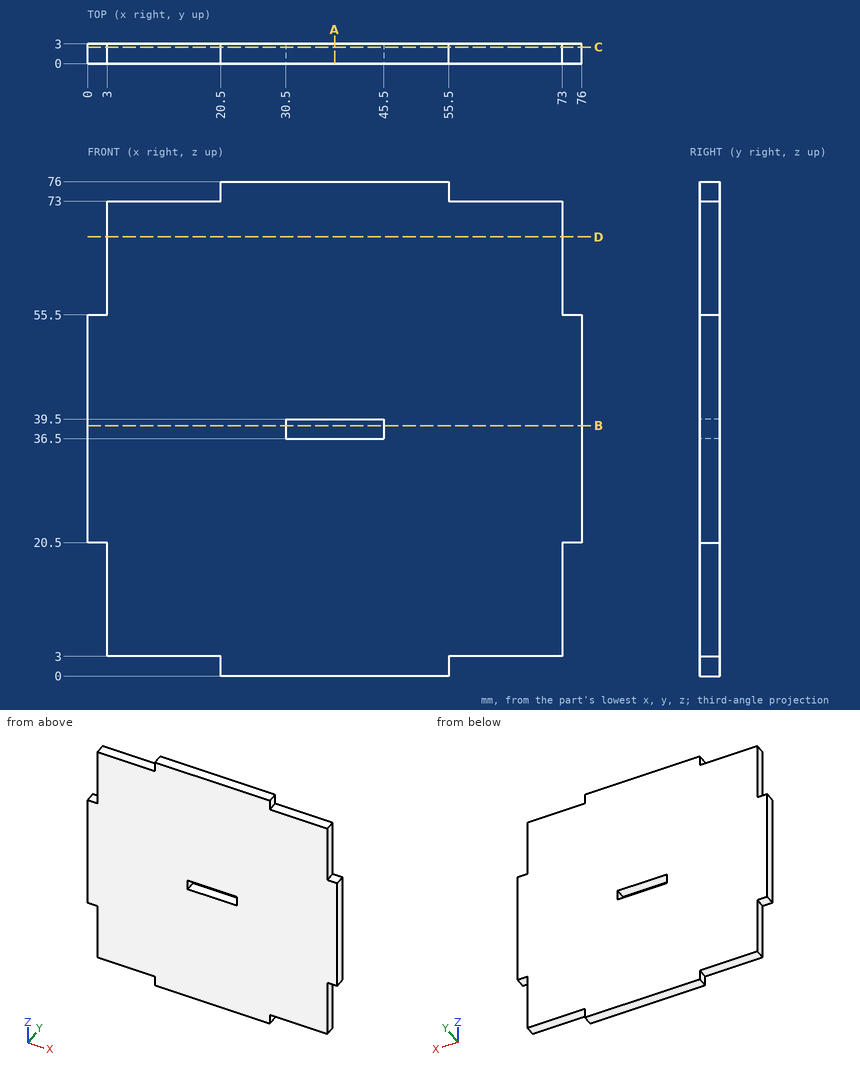
The figure shows three views and two pictorial views of one solid part (mm, origin at its lowest corner). Answer the questions. Give positions to 0.01 mm unless a question says otherwise; leave off trailing zeros. Order: outer loops, then holes, each group sorted by start corner. A loop starts at its lowest first (then second) coordinate and runs counter-clockwise, first axis right, second up. Notation, with made-up numbers: (57, 36.25) -> (95, 36.25) arc R17 ccw to (95, 49.25) -> close; hole circle Ø4 at (-4.75, 19.25). An arc over 180 degrees is marked (long way). Answer as a JSON object with one key per item and string values. Group by question number.
Item 1: The part is cut by section B-B on z = 38.5. Write down the section's boundary in (x, y), and give its area (3 significant figures).
Item 2: The part is cut by section D-D on z = 67.5. Write down the section's boundary in (x, y), and give its area (3 significant figures).
Item 3: The part is cut by section C-C on y = 2.5. Write down the section's boundary in (x, z).
Item 4: Flat-ended cylindrical pins translate along their axes: pin 1 (1.5 mm diameter, centred on y = 1.5, z = 1.5, fed in from +X); pin 2 (1.5 mm diameter, centred on y = 1.5, z = 9, fed in from -X); pin 3 (1.5 mm diameter, centred on x = 22.5, y = 0.5, fed in from -Z); pin 4 (0.9 mm diameter, centred on x = 74, y = 1, fed in from -Z). Find the tip coordinate at first contact, or state that the pin passes through.
Item 5: Consider L1, parallel to Z at x = 43.5, y = 1.6; L2, parallel to X at y = 1.6, z = 20. Determine where each line is inside the solid, lowest interval first. Write a range as from..to.
Item 6: The part is cut by section A-A on x = 38. Write down the section's boundary in (y, z).
Result set:
{
 "1": {"outline": "(0, 0) -> (30.5, 0) -> (30.5, 3) -> (0, 3) -> close; (45.5, 0) -> (76, 0) -> (76, 3) -> (45.5, 3) -> close", "area": "183 mm²"},
 "2": {"outline": "(3, 0) -> (73, 0) -> (73, 3) -> (3, 3) -> close", "area": "210 mm²"},
 "3": {"outline": "(0, 20.5) -> (3, 20.5) -> (3, 3) -> (20.5, 3) -> (20.5, 0) -> (55.5, 0) -> (55.5, 3) -> (73, 3) -> (73, 20.5) -> (76, 20.5) -> (76, 55.5) -> (73, 55.5) -> (73, 73) -> (55.5, 73) -> (55.5, 76) -> (20.5, 76) -> (20.5, 73) -> (3, 73) -> (3, 55.5) -> (0, 55.5) -> close; hole (30.5, 36.5) -> (45.5, 36.5) -> (45.5, 39.5) -> (30.5, 39.5) -> close"},
 "4": {"pin 1": "x = 55.5", "pin 2": "x = 3", "pin 3": "z = 0", "pin 4": "z = 20.5"},
 "5": {"L1": "0..36.5, 39.5..76", "L2": "3..73"},
 "6": {"outline": "(0, 0) -> (3, 0) -> (3, 36.5) -> (0, 36.5) -> close; (0, 39.5) -> (3, 39.5) -> (3, 76) -> (0, 76) -> close"}
}
